Source: CAD feature listing. Evaluate the final solid. Frame: model axes, mm. Give positions to 0.01 mm unless a question says otherwise; leave off trailing zeros. Answer as a JSON object with one key per item and string values. Group by question number.
from build123d import *

# Parameters (mm, degrees)
SKETCH1_R           = 275
BOSS_EXTRUDE1_DEPTH = 5


with BuildPart() as part:
    # Sketch1 → Boss-Extrude1 (new body)
    with BuildSketch(Plane(origin=(0, 0, 0), x_dir=(1, 0, 0), z_dir=(0, 1, 0))):
        with Locations(Location((0, 0, 0), (0, 0, 270))):
            Circle(SKETCH1_R)
        with BuildLine():
            Line((269.988425678, 2.5), (-269.988425678, 2.5))
            ThreePointArc((-269.988425678, 2.5), (-269.814607969, 10.003865569), (-269.432273494, 17.5))
            Line((-269.432273494, 17.5), (269.432273494, 17.5))
            ThreePointArc((269.432273494, 17.5), (269.814607969, 10.003865569), (269.988425678, 2.5))
        make_face(mode=Mode.SUBTRACT)
        with BuildLine():
            Line((-269.988425678, -2.5), (269.988425678, -2.5))
            ThreePointArc((269.988425678, -2.5), (269.814607969, -10.003865569), (269.432273494, -17.5))
            Line((269.432273494, -17.5), (-269.432273494, -17.5))
            ThreePointArc((-269.432273494, -17.5), (-269.814607969, -10.003865569), (-269.988425678, -2.5))
        make_face(mode=Mode.SUBTRACT)
        with BuildLine():
            ThreePointArc((267.38315205, 37.5), (268.326846063, 30.011725736), (269.06086672, 22.5))
            Line((269.06086672, 22.5), (-269.06086672, 22.5))
            ThreePointArc((-269.06086672, 22.5), (-268.326846063, 30.011725736), (-267.38315205, 37.5))
            Line((-267.38315205, 37.5), (267.38315205, 37.5))
        make_face(mode=Mode.SUBTRACT)
        with BuildLine():
            ThreePointArc((263.806273618, 57.5), (265.326215877, 50.019987688), (266.634112596, 42.5))
            Line((266.634112596, 42.5), (-266.634112596, 42.5))
            ThreePointArc((-266.634112596, 42.5), (-265.326215877, 50.019987688), (-263.806273618, 57.5))
            Line((-263.806273618, 57.5), (263.806273618, 57.5))
        make_face(mode=Mode.SUBTRACT)
        with BuildLine():
            ThreePointArc((258.638260897, 77.5), (260.760317328, 70.02897191), (262.66661379, 62.5))
            Line((262.66661379, 62.5), (-262.66661379, 62.5))
            ThreePointArc((-262.66661379, 62.5), (-260.760317328, 70.02897191), (-258.638260897, 77.5))
            Line((-258.638260897, 77.5), (258.638260897, 77.5))
        make_face(mode=Mode.SUBTRACT)
        with BuildLine():
            ThreePointArc((251.781154974, 97.5), (254.544616671, 90.039092198), (257.087047515, 82.5))
            Line((257.087047515, 82.5), (-257.087047515, 82.5))
            ThreePointArc((-257.087047515, 82.5), (-254.544616671, 90.039092198), (-251.781154974, 97.5))
            Line((-251.781154974, 97.5), (251.781154974, 97.5))
        make_face(mode=Mode.SUBTRACT)
        with BuildLine():
            ThreePointArc((243.092060751, 117.5), (246.553834032, 110.050928774), (249.787409611, 102.5))
            Line((249.787409611, 102.5), (-249.787409611, 102.5))
            ThreePointArc((-249.787409611, 102.5), (-246.553834032, 110.050928774), (-243.092060751, 117.5))
            Line((-243.092060751, 117.5), (243.092060751, 117.5))
        make_face(mode=Mode.SUBTRACT)
        with BuildLine():
            ThreePointArc((232.365552524, 137.5), (236.607274446, 130.065359259), (240.611200903, 122.5))
            Line((240.611200903, 122.5), (-240.611200903, 122.5))
            ThreePointArc((-240.611200903, 122.5), (-236.607274446, 130.065359259), (-232.365552524, 137.5))
            Line((-232.365552524, 137.5), (232.365552524, 137.5))
        make_face(mode=Mode.SUBTRACT)
        with BuildLine():
            ThreePointArc((219.302872758, 157.5), (224.443417745, 150.083817353), (229.333272771, 142.5))
            Line((229.333272771, 142.5), (-229.333272771, 142.5))
            ThreePointArc((-229.333272771, 142.5), (-224.443417745, 150.083817353), (-219.302872758, 157.5))
            Line((-219.302872758, 157.5), (219.302872758, 157.5))
        make_face(mode=Mode.SUBTRACT)
        with BuildLine():
            ThreePointArc((203.454540377, 177.5), (209.673497347, 170.108860763), (215.624094201, 162.5))
            Line((215.624094201, 162.5), (-215.624094201, 162.5))
            ThreePointArc((-215.624094201, 162.5), (-209.673497347, 170.108860763), (-203.454540377, 177.5))
            Line((-203.454540377, 177.5), (203.454540377, 177.5))
        make_face(mode=Mode.SUBTRACT)
        with BuildLine():
            ThreePointArc((184.102552943, 197.5), (191.688946284, 190.145596511), (198.981783086, 182.5))
            Line((198.981783086, 182.5), (-198.981783086, 182.5))
            ThreePointArc((-198.981783086, 182.5), (-191.688946284, 190.145596511), (-184.102552943, 197.5))
            Line((-184.102552943, 197.5), (184.102552943, 197.5))
        make_face(mode=Mode.SUBTRACT)
        with BuildLine():
            ThreePointArc((159.980467558, 217.5), (169.450399668, 210.205999087), (178.588213497, 202.5))
            Line((178.588213497, 202.5), (-178.588213497, 202.5))
            ThreePointArc((-178.588213497, 202.5), (-169.450399668, 210.205999087), (-159.980467558, 217.5))
            Line((-159.980467558, 217.5), (159.980467558, 217.5))
        make_face(mode=Mode.SUBTRACT)
        with BuildLine():
            ThreePointArc((128.42799539, 237.5), (140.888842421, 230.326581361), (152.950155279, 222.5))
            Line((152.950155279, 222.5), (-152.950155279, 222.5))
            ThreePointArc((-152.950155279, 222.5), (-140.888842421, 230.326581361), (-128.42799539, 237.5))
            Line((-128.42799539, 237.5), (128.42799539, 237.5))
        make_face(mode=Mode.SUBTRACT)
        with BuildLine():
            ThreePointArc((81.201908845, 257.5), (100.240473836, 250.702707215), (118.717100706, 242.5))
            Line((118.717100706, 242.5), (-118.717100706, 242.5))
            ThreePointArc((-118.717100706, 242.5), (-100.240473836, 250.702707215), (-81.201908845, 257.5))
            Line((-81.201908845, 257.5), (81.201908845, 257.5))
        make_face(mode=Mode.SUBTRACT)
        with BuildLine():
            ThreePointArc((269.06086672, -22.5), (268.326846063, -30.011725736), (267.38315205, -37.5))
            Line((267.38315205, -37.5), (-267.38315205, -37.5))
            ThreePointArc((-267.38315205, -37.5), (-268.326846063, -30.011725736), (-269.06086672, -22.5))
            Line((-269.06086672, -22.5), (269.06086672, -22.5))
        make_face(mode=Mode.SUBTRACT)
        with BuildLine():
            ThreePointArc((-263.806273618, -57.5), (-265.326215877, -50.019987688), (-266.634112596, -42.5))
            Line((-266.634112596, -42.5), (266.634112596, -42.5))
            ThreePointArc((266.634112596, -42.5), (265.326215877, -50.019987688), (263.806273618, -57.5))
            Line((263.806273618, -57.5), (-263.806273618, -57.5))
        make_face(mode=Mode.SUBTRACT)
        with BuildLine():
            ThreePointArc((-258.638260897, -77.5), (-260.760317328, -70.02897191), (-262.66661379, -62.5))
            Line((-262.66661379, -62.5), (262.66661379, -62.5))
            ThreePointArc((262.66661379, -62.5), (260.760317328, -70.02897191), (258.638260897, -77.5))
            Line((258.638260897, -77.5), (-258.638260897, -77.5))
        make_face(mode=Mode.SUBTRACT)
        with BuildLine():
            ThreePointArc((-251.781154974, -97.5), (-254.544616671, -90.039092198), (-257.087047515, -82.5))
            Line((-257.087047515, -82.5), (257.087047515, -82.5))
            ThreePointArc((257.087047515, -82.5), (254.544616671, -90.039092198), (251.781154974, -97.5))
            Line((251.781154974, -97.5), (-251.781154974, -97.5))
        make_face(mode=Mode.SUBTRACT)
        with BuildLine():
            ThreePointArc((-243.092060751, -117.5), (-246.553834032, -110.050928774), (-249.787409611, -102.5))
            Line((-249.787409611, -102.5), (249.787409611, -102.5))
            ThreePointArc((249.787409611, -102.5), (246.553834032, -110.050928774), (243.092060751, -117.5))
            Line((243.092060751, -117.5), (-243.092060751, -117.5))
        make_face(mode=Mode.SUBTRACT)
        with BuildLine():
            ThreePointArc((-232.365552524, -137.5), (-236.607274446, -130.065359259), (-240.611200903, -122.5))
            Line((-240.611200903, -122.5), (240.611200903, -122.5))
            ThreePointArc((240.611200903, -122.5), (236.607274446, -130.065359259), (232.365552524, -137.5))
            Line((232.365552524, -137.5), (-232.365552524, -137.5))
        make_face(mode=Mode.SUBTRACT)
        with BuildLine():
            ThreePointArc((-219.302872758, -157.5), (-224.443417745, -150.083817353), (-229.333272771, -142.5))
            Line((-229.333272771, -142.5), (229.333272771, -142.5))
            ThreePointArc((229.333272771, -142.5), (224.443417745, -150.083817353), (219.302872758, -157.5))
            Line((219.302872758, -157.5), (-219.302872758, -157.5))
        make_face(mode=Mode.SUBTRACT)
        with BuildLine():
            ThreePointArc((-203.454540377, -177.5), (-209.673497347, -170.108860763), (-215.624094201, -162.5))
            Line((-215.624094201, -162.5), (215.624094201, -162.5))
            ThreePointArc((215.624094201, -162.5), (209.673497347, -170.108860763), (203.454540377, -177.5))
            Line((203.454540377, -177.5), (-203.454540377, -177.5))
        make_face(mode=Mode.SUBTRACT)
        with BuildLine():
            ThreePointArc((-184.102552943, -197.5), (-191.688946284, -190.145596511), (-198.981783086, -182.5))
            Line((-198.981783086, -182.5), (198.981783086, -182.5))
            ThreePointArc((198.981783086, -182.5), (191.688946284, -190.145596511), (184.102552943, -197.5))
            Line((184.102552943, -197.5), (-184.102552943, -197.5))
        make_face(mode=Mode.SUBTRACT)
        with BuildLine():
            ThreePointArc((-159.980467558, -217.5), (-169.450399668, -210.205999087), (-178.588213497, -202.5))
            Line((-178.588213497, -202.5), (178.588213497, -202.5))
            ThreePointArc((178.588213497, -202.5), (169.450399668, -210.205999087), (159.980467558, -217.5))
            Line((159.980467558, -217.5), (-159.980467558, -217.5))
        make_face(mode=Mode.SUBTRACT)
        with BuildLine():
            ThreePointArc((-128.42799539, -237.5), (-140.888842421, -230.326581361), (-152.950155279, -222.5))
            Line((-152.950155279, -222.5), (152.950155279, -222.5))
            ThreePointArc((152.950155279, -222.5), (140.888842421, -230.326581361), (128.42799539, -237.5))
            Line((128.42799539, -237.5), (-128.42799539, -237.5))
        make_face(mode=Mode.SUBTRACT)
        with BuildLine():
            ThreePointArc((-81.201908845, -257.5), (-100.240473836, -250.702707215), (-118.717100706, -242.5))
            Line((-118.717100706, -242.5), (118.717100706, -242.5))
            ThreePointArc((118.717100706, -242.5), (100.240473836, -250.702707215), (81.201908845, -257.5))
            Line((81.201908845, -257.5), (-81.201908845, -257.5))
        make_face(mode=Mode.SUBTRACT)
    extrude(amount=BOSS_EXTRUDE1_DEPTH)


solid = part.part
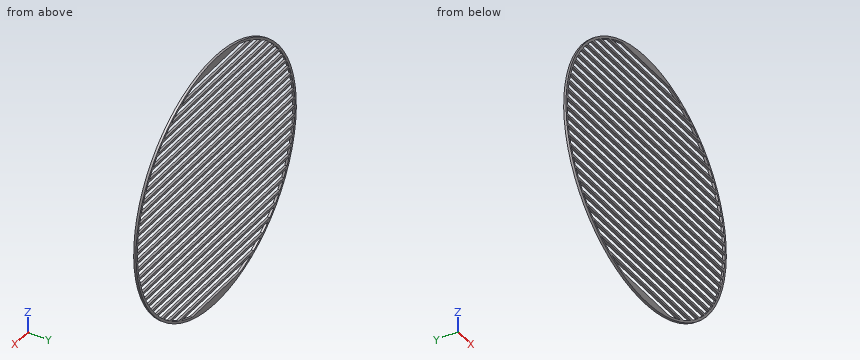
(1) Material intervals for line 1 (X direction, y = 0.2, z = -4.5); line 2 (X direction, y = 2.9, z = -37); line 3 (X direction, y = 4, z = -138.5), sorted ascending. Write a range as from..to.
(2) First-contact query: pin 1 (1.5 mm diameter, centred on x = -186, y = 4, fed in from -Z); pin 2 (1.5 mm diameter, centred on x = -108.5, y = 3.5, fed in from +Z); pin 3 (2.5 mm diameter, centred on x = 37, y = 3, fed in from +Z). Flat tips, straight axial feed; report the tip coordinate or a pass-through.
(3) Section query A-A on x = 0. State how many separate pieces and enclosed holes the cut face has, plus the area to 3 significant figures.
Result:
{
 "1": {"line 1": "-274.96..-269.96, 269.96..274.96", "line 2": "-272.5..-267.45, 267.45..272.5", "line 3": "-237.58..237.58"},
 "2": {"pin 1": "z = -203.24", "pin 2": "z = 253.01", "pin 3": "z = 272.67"},
 "3": {"separate pieces": "27", "enclosed holes": "0", "area": "800 mm²"}
}
